The model under review builds one solid part; all positions refer to its coordinate system, in mm. Face numbers are marked on the shaded views. Give positions to 0.01 mm unless a question says otherwise; leave off trailing zeros. Order: outer loops, then holes, each group sorted by start corner. A loop starts at its lowest first (then second) coordinate and runs counter-clockwise, first axis right, second up. Notation, with made-up numbers: (48, 22.25) - (55, 22.25) arc R28 cw to (55, 50.25) - close; hole circle Ø8 at (88, -24.5). An arc over 180 degrees is marked (long way). Use CSV: the item, a comma, the result in double quotes.
```python
from build123d import *

# Parameters (mm, degrees)
F1_DEPTH = 1.5
F2_W     = 74.9872508645
F2_H     = 97.9872508645
F2_W_2   = 70.9872508645
F2_H_2   = 93.9872508645
F3_DEPTH = 5
F4_W     = 8
F4_H     = 8
F4_R     = 1.3
F5_DEPTH = 3.4
F6_R     = 2


with BuildPart() as f1:
    # F0 (on Top) → F1 (new body)
    with BuildSketch(Plane.XY):
        Polygon((-39.4936254323, -50.4936254323), (-37, -50.4936254323), (33, -50.4936254323), (35.4936254323, -50.4936254323), (35.4936254323, -48), (35.4936254323, 45), (35.4936254323, 47.4936254323), (33, 47.4936254323), (-37, 47.4936254323), (-39.4936254323, 47.4936254323), (-39.4936254323, -47.5), align=None)
    extrude(amount=F1_DEPTH)

    # F2 (on face) → F3 (join)
    with BuildSketch(Plane.XY.offset(1.5)):
        with Locations((-2, -1.5)):
            Rectangle(F2_W, F2_H)
        with Locations((-2, -1.5)):
            Rectangle(F2_W_2, F2_H_2, mode=Mode.SUBTRACT)
    extrude(amount=F3_DEPTH)

    # F4 (on face) → F5 (join)
    with BuildSketch(Plane.XY.offset(1.5)):
        with Locations((-33.4936254323, 41.4936254323)):
            Rectangle(F4_W, F4_H)
        with Locations((-32.9936254323, 40.9936254323)):
            Circle(F4_R, mode=Mode.SUBTRACT)
        with Locations((29.4936254323, 41.4936254323)):
            Rectangle(F4_W, F4_H)
        with Locations((28.9936254323, 40.9936254323)):
            Circle(F4_R, mode=Mode.SUBTRACT)
        with Locations((29.4936254323, -44.4936254323)):
            Rectangle(F4_W, F4_H)
        with Locations((28.9936254323, -43.9936254323)):
            Circle(F4_R, mode=Mode.SUBTRACT)
        with Locations((-33.4936254323, -44.4936254323)):
            Rectangle(F4_W, F4_H)
        with Locations((-32.9936254323, -43.9936254323)):
            Circle(F4_R, mode=Mode.SUBTRACT)
    extrude(amount=F5_DEPTH)

    # F6
    f6_edges = [f1.edges().sort_by_distance(p)[0] for p in [
        (-39.493625, -50.493625, 3.25),
        (-39.493625, 47.493625, 3.25),
        (35.493625, 47.493625, 3.25),
        (35.493625, -50.493625, 3.25),
    ]]
    fillet(f6_edges, radius=F6_R)


solid = f1.part
```
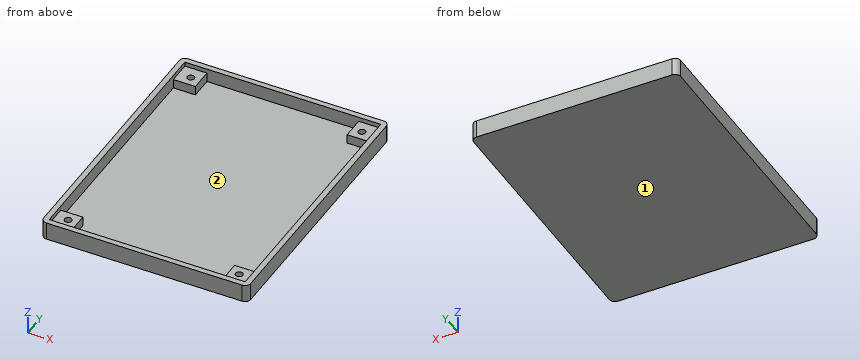
Item 1: Clearance check with flat-ended pins moving along their axes: pin 1 (2.5 mm diameter, centred on x = 29.5, y = -43, fed in from +Z); pin 2 (1.6 mm diameter, centred on x = 28.99, y = 40.99, fed in from +Z). State where each tip first meets the part, or that it passes through.
Results list:
pin 1,"stops at z = 4.9"
pin 2,"stops at z = 1.5"
Item 2: Take a section at A-A, the plane x = 22. Give the boundary of the cut face in (y, z), and give its area (3 significant figures).
Results list:
outline,"(-50.49, 0) - (47.49, 0) - (47.49, 6.5) - (45.49, 6.5) - (45.49, 1.5) - (-48.49, 1.5) - (-48.49, 6.5) - (-50.49, 6.5) - close"
area,"167 mm2"
Item 3: Wall thickness on L1, parallel to X at y = -13, z = 6; L2, parallel to Y at x = -22, z = 4.5; L3, parallel to Y at x = 32, z = 3.5: over which ranges is each line inside the solid? List them lowest first.
Results list:
L1,"x = -39.49 to -37.49, 33.49 to 35.49"
L2,"y = -50.49 to -48.49, 45.49 to 47.49"
L3,"y = -50.49 to -40.49, 37.49 to 47.49"
Item 4: Take a section at C-C, the plane z = 2.75. Give the boundary of the cut face in (x, y), and give its area (3 significant figures).
Results list:
outline,"(-39.49, -48.49) arc R2 ccw to (-37.49, -50.49) - (33.49, -50.49) arc R2 ccw to (35.49, -48.49) - (35.49, 45.49) arc R2 ccw to (33.49, 47.49) - (-37.49, 47.49) arc R2 ccw to (-39.49, 45.49) - close; hole (-37.49, -40.49) - (-29.49, -40.49) - (-29.49, -48.49) - (25.49, -48.49) - (25.49, -40.49) - (33.49, -40.49) - (33.49, 37.49) - (25.49, 37.49) - (25.49, 45.49) - (-29.49, 45.49) - (-29.49, 37.49) - (-37.49, 37.49) - close; hole circle Ø2.6 at (-32.99, -43.99); hole circle Ø2.6 at (-32.99, 40.99); hole circle Ø2.6 at (28.99, -43.99); hole circle Ø2.6 at (28.99, 40.99)"
area,"907 mm2"
Item 5: Take a section at B-B, the plane y = -25.5. Give the boundary of the cut face in (x, z), and give its area (3 significant figures).
Results list:
outline,"(-39.49, 0) - (35.49, 0) - (35.49, 6.5) - (33.49, 6.5) - (33.49, 1.5) - (-37.49, 1.5) - (-37.49, 6.5) - (-39.49, 6.5) - close"
area,"132 mm2"
Item 6: Mouldability with a two-part tool opening along Y and no side actions: class the marked faces 1 and 2 as pulls with the +Y half, pulls with the -Y half, needs draft (parallel to the pull), parting line crosses it, or undercut.
Results list:
face 1,"needs draft"
face 2,"undercut"
